Answer from the drawing. Dimensions are ordinates in mm from the lowest x, y and z of the part. Give positions to 0.01 mm unless a question says otherwise; leave off trailing zeros. Order: outer loops, then holes, each group sorted by start corner. A loop starts at its lowest first (then second) coordinate and runs counter-clockwise, first axis right, second up. Notation, with made-up numbers: (17, 44) - (31, 44) arc R32 cw to (31, 78) - close; hole circle Ø2 at (38.25, 88). An arc over 180 degrees is marked (long way). Write each question's results on one line, items separated by ' | '.
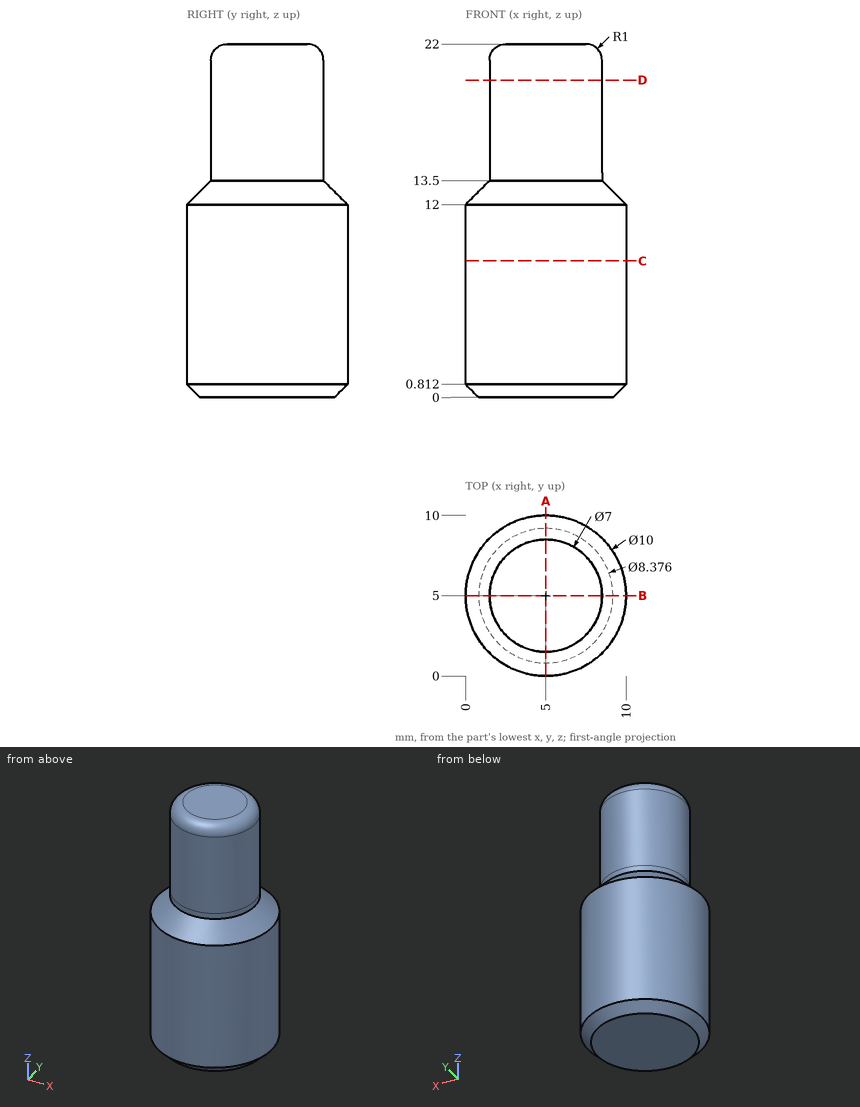
(1) Section D-D (z = 19.75) is taken. Give the vertices of the cut face in (x, y).
Conclusion:
outline: circle Ø7 at (5, 5)
(2) Section A-A (x = 5) is taken. Give the vertices of the cut face in (y, z).
Conclusion:
outline: (0, 0.81) - (0.81, 0) - (9.19, 0) - (10, 0.81) - (10, 12) - (8.5, 13.5) - (8.5, 21) arc R1 ccw to (7.5, 22) - (2.5, 22) arc R1 ccw to (1.5, 21) - (1.5, 13.5) - (0, 12) - close
(3) Consider probe 1 along Z at (x, y) = (3.25, 1.25); probe 2 along Y at (x, z) = (4.75, 8.25); probe 3 along Y at (x, z) = (1.25, 1). Determine where each line is inside the solid, lowest interval first. Write a range as [from, to].
Conclusion:
probe 1: [0, 12.86] | probe 2: [0.01, 9.99] | probe 3: [1.69, 8.31]
(4) This flat-tipped pin is pushed along its axis until it touches: pin 1 (5 mm diameter, centred on x = 8.5, z = 18.5, fed in from +Y). Where does it stop, or does it pass through?
Conclusion:
pin 1: y = 8.35
(5) Section C-C (z = 8.5) is taken. Give the vertices of the cut face in (x, y), plus the area to 3 significant figures.
Conclusion:
outline: circle Ø10 at (5, 5) | area: 78.5 mm^2
